```python
from build123d import *

# Parameters (mm, degrees)
SKETCH1_R              = 1.651
SKETCH1_R_2            = 1.8415
SKETCH1_R_3            = 1.905
SKETCH1_R_4            = 3.175
SKETCH1_R_5            = 1.315256363
SKETCH1_R_6            = 1.5621
SKETCH1_R_7            = 5.08
SKETCH1_R_8            = 2.2479
BOSS_EXTRUDE1_DEPTH    = 6.35
FILLET_OUTER_CORNERS_R = 12.7
FILLET_INNER_CORNERS_R = 6.35
SKETCH2_R              = 5.08
CUT_EXTRUDE1_DEPTH     = 220.86103505


with BuildPart() as part:
    # Sketch1 → Boss-Extrude1 (new body)
    with BuildSketch(Plane(origin=(0, 0, 0), x_dir=(1, 0, 0), z_dir=(0, 1, 0))):
        with BuildLine():
            Line((-142.875, 95.25), (-41.275, 95.25))
            Line((-41.275, 95.25), (-41.275, 139.7))
            Line((-41.275, 139.7), (41.275, 139.7))
            Line((41.275, 139.7), (41.275, 95.25))
            Line((41.275, 95.25), (142.875, 95.25))
            Line((142.875, 95.25), (170.571792564, 95.25))
            ThreePointArc((170.571792564, 95.25), (166.994880438, 0), (170.571792564, -95.25))
            Line((170.571792564, -95.25), (142.875, -95.25))
            Line((142.875, -95.25), (41.275, -95.25))
            Line((41.275, -95.25), (41.275, -139.7))
            Line((41.275, -139.7), (-41.275, -139.7))
            Line((-41.275, -139.7), (-41.275, -95.25))
            Line((-41.275, -95.25), (-142.875, -95.25))
            Line((-142.875, -95.25), (-170.571792564, -95.25))
            ThreePointArc((-170.571792564, -95.25), (-166.994880438, 0), (-170.571792564, 95.25))
            Line((-170.571792564, 95.25), (-142.875, 95.25))
        make_face()
        with Locations(Location((-107.696, 77.978, 0), (0, 0, 270))):
            Circle(SKETCH1_R, mode=Mode.SUBTRACT)
        with Locations(Location((-107.696, 65.278, 0), (0, 0, 270))):
            Circle(SKETCH1_R, mode=Mode.SUBTRACT)
        with Locations(Location((-107.696, 52.578, 0), (0, 0, 270))):
            Circle(SKETCH1_R, mode=Mode.SUBTRACT)
        with Locations(Location((-76.454, 77.978, 0), (0, 0, 90))):
            Circle(SKETCH1_R, mode=Mode.SUBTRACT)
        with Locations(Location((-76.454, 65.278, 0), (0, 0, 90))):
            Circle(SKETCH1_R, mode=Mode.SUBTRACT)
        with Locations(Location((-76.454, 52.578, 0), (0, 0, 90))):
            Circle(SKETCH1_R, mode=Mode.SUBTRACT)
        with Locations(Location((76.454, 52.578, 0), (0, 0, 270))):
            Circle(SKETCH1_R, mode=Mode.SUBTRACT)
        with Locations(Location((107.696, 52.578, 0), (0, 0, 90))):
            Circle(SKETCH1_R, mode=Mode.SUBTRACT)
        with Locations(Location((76.454, 65.278, 0), (0, 0, 270))):
            Circle(SKETCH1_R, mode=Mode.SUBTRACT)
        with Locations(Location((107.696, 65.278, 0), (0, 0, 90))):
            Circle(SKETCH1_R, mode=Mode.SUBTRACT)
        with Locations(Location((76.454, 77.978, 0), (0, 0, 270))):
            Circle(SKETCH1_R, mode=Mode.SUBTRACT)
        with Locations(Location((107.696, 77.978, 0), (0, 0, 90))):
            Circle(SKETCH1_R, mode=Mode.SUBTRACT)
        with Locations(Location((76.454, -52.578, 0), (0, 0, 90))):
            Circle(SKETCH1_R, mode=Mode.SUBTRACT)
        with Locations(Location((107.696, -52.578, 0), (0, 0, 270))):
            Circle(SKETCH1_R, mode=Mode.SUBTRACT)
        with Locations(Location((107.696, -65.278, 0), (0, 0, 270))):
            Circle(SKETCH1_R, mode=Mode.SUBTRACT)
        with Locations(Location((76.454, -65.278, 0), (0, 0, 90))):
            Circle(SKETCH1_R, mode=Mode.SUBTRACT)
        with Locations(Location((107.696, -77.978, 0), (0, 0, 270))):
            Circle(SKETCH1_R, mode=Mode.SUBTRACT)
        with Locations(Location((76.454, -77.978, 0), (0, 0, 90))):
            Circle(SKETCH1_R, mode=Mode.SUBTRACT)
        with Locations(Location((-76.454, -52.578, 0), (0, 0, 270))):
            Circle(SKETCH1_R, mode=Mode.SUBTRACT)
        with Locations(Location((-107.696, -52.578, 0), (0, 0, 90))):
            Circle(SKETCH1_R, mode=Mode.SUBTRACT)
        with Locations(Location((-76.454, -65.278, 0), (0, 0, 270))):
            Circle(SKETCH1_R, mode=Mode.SUBTRACT)
        with Locations(Location((-107.696, -65.278, 0), (0, 0, 90))):
            Circle(SKETCH1_R, mode=Mode.SUBTRACT)
        with Locations(Location((-76.454, -77.978, 0), (0, 0, 270))):
            Circle(SKETCH1_R, mode=Mode.SUBTRACT)
        with Locations(Location((-107.696, -77.978, 0), (0, 0, 90))):
            Circle(SKETCH1_R, mode=Mode.SUBTRACT)
        with Locations(Location((155.575, 0, 0), (0, 0, 270))):
            Circle(SKETCH1_R_2, mode=Mode.SUBTRACT)
        with Locations(Location((-27.94, -128.27, 0), (0, 0, 270))):
            Circle(SKETCH1_R_3, mode=Mode.SUBTRACT)
        with Locations(Location((27.94, -128.27, 0), (0, 0, 270))):
            Circle(SKETCH1_R_3, mode=Mode.SUBTRACT)
        with Locations(Location((-27.94, -41.91, 0), (0, 0, 90))):
            Circle(SKETCH1_R_3, mode=Mode.SUBTRACT)
        with Locations(Location((27.94, -41.91, 0), (0, 0, 90))):
            Circle(SKETCH1_R_3, mode=Mode.SUBTRACT)
        with Locations(Location((0, 0, 0), (0, 0, 270))):
            Circle(SKETCH1_R_2, mode=Mode.SUBTRACT)
        with Locations(Location((-122.311792564, 69.85, 0), (0, 0, 270))):
            Circle(SKETCH1_R_4, mode=Mode.SUBTRACT)
        with Locations(Location((-61.838207436, 69.85, 0), (0, 0, 90))):
            Circle(SKETCH1_R_4, mode=Mode.SUBTRACT)
        with Locations(Location((-61.838207436, -69.85, 0), (0, 0, 270))):
            Circle(SKETCH1_R_4, mode=Mode.SUBTRACT)
        with Locations(Location((-122.311792564, -69.85, 0), (0, 0, 90))):
            Circle(SKETCH1_R_4, mode=Mode.SUBTRACT)
        with Locations(Location((61.838207436, -69.85, 0), (0, 0, 90))):
            Circle(SKETCH1_R_4, mode=Mode.SUBTRACT)
        with Locations(Location((122.311792564, -69.85, 0), (0, 0, 270))):
            Circle(SKETCH1_R_4, mode=Mode.SUBTRACT)
        with Locations(Location((61.838207436, 69.85, 0), (0, 0, 270))):
            Circle(SKETCH1_R_4, mode=Mode.SUBTRACT)
        with Locations(Location((122.311792564, 69.85, 0), (0, 0, 90))):
            Circle(SKETCH1_R_4, mode=Mode.SUBTRACT)
        with Locations(Location((149.480692766, -14.9479, 0), (0, 0, 270))):
            Circle(SKETCH1_R_5, mode=Mode.SUBTRACT)
        with Locations(Location((121.464492766, -14.9479, 0), (0, 0, 270))):
            Circle(SKETCH1_R_6, mode=Mode.SUBTRACT)
        with Locations(Location((116.586, -45.9486, 0), (0, 0, 270))):
            Circle(SKETCH1_R_6, mode=Mode.SUBTRACT)
        with Locations(Location((164.9222, -38.4556, 0), (0, 0, 270))):
            Circle(SKETCH1_R_6, mode=Mode.SUBTRACT)
        with Locations(Location((164.9222, 36.6776, 0), (0, 0, 270))):
            Circle(SKETCH1_R_6, mode=Mode.SUBTRACT)
        with Locations(Location((116.586, 36.6776, 0), (0, 0, 270))):
            Circle(SKETCH1_R_6, mode=Mode.SUBTRACT)
        with Locations(Location((0, -92.075, 0), (0, 0, 270))):
            Circle(SKETCH1_R_3, mode=Mode.SUBTRACT)
        with Locations(Location((0, 92.075, 0), (0, 0, 270))):
            Circle(SKETCH1_R_3, mode=Mode.SUBTRACT)
        with Locations(Location((-61.838207436, -39.878, 0), (0, 0, 270))):
            Circle(SKETCH1_R_7, mode=Mode.SUBTRACT)
        with Locations(Location((-122.311792564, -39.878, 0), (0, 0, 270))):
            Circle(SKETCH1_R_7, mode=Mode.SUBTRACT)
        with Locations(Location((61.838207436, -39.878, 0), (0, 0, 90))):
            Circle(SKETCH1_R_7, mode=Mode.SUBTRACT)
        with Locations(Location((62.026925824, -8.128150569, 0), (0, 0, 270))):
            Circle(SKETCH1_R_8, mode=Mode.SUBTRACT)
        with Locations(Location((64.176925824, 48.924363993, 0), (0, 0, 270))):
            Circle(SKETCH1_R_8, mode=Mode.SUBTRACT)
        with Locations(Location((64.176925824, 55.924363993, 0), (0, 0, 270))):
            Circle(SKETCH1_R_8, mode=Mode.SUBTRACT)
        with Locations(Location((-33.323074176, 55.924363993, 0), (0, 0, 270))):
            Circle(SKETCH1_R_8, mode=Mode.SUBTRACT)
        with Locations(Location((-33.323074176, 48.924363993, 0), (0, 0, 270))):
            Circle(SKETCH1_R_8, mode=Mode.SUBTRACT)
        with Locations(Location((-39.573074176, 0.761849431, 0), (0, 0, 270))):
            Circle(SKETCH1_R_8, mode=Mode.SUBTRACT)
        with Locations(Location((-84.023074176, 0.761849431, 0), (0, 0, 270))):
            Circle(SKETCH1_R_8, mode=Mode.SUBTRACT)
        with Locations(Location((-128.473074176, 0.761849431, 0), (0, 0, 270))):
            Circle(SKETCH1_R_8, mode=Mode.SUBTRACT)
    extrude(amount=BOSS_EXTRUDE1_DEPTH)

    # Fillet_Outer_Corners
    fillet_outer_corners_edges = [part.edges().sort_by_distance(p)[0] for p in [
        (-170.571792564, 3.175, 95.25),
        (-170.571792564, 3.175, -95.25),
        (-41.275, 3.175, -139.7),
        (41.275, 3.175, -139.7),
        (170.571792564, 3.175, -95.25),
        (170.571792564, 3.175, 95.25),
        (41.275, 3.175, 139.7),
        (-41.275, 3.175, 139.7),
    ]]
    fillet(fillet_outer_corners_edges, radius=FILLET_OUTER_CORNERS_R)

    # Fillet_Inner_Corners
    fillet_inner_corners_edges = [part.edges().sort_by_distance(p)[0] for p in [
        (-41.275, 3.175, -95.25),
        (41.275, 3.175, -95.25),
        (41.275, 3.175, 95.25),
        (-41.275, 3.175, 95.25),
    ]]
    fillet(fillet_inner_corners_edges, radius=FILLET_INNER_CORNERS_R)

    # Sketch2 → Cut-Extrude1 (cut, through all)
    with BuildSketch(Plane(origin=(0, 6.35, 0), x_dir=(1, 0, 0), z_dir=(0, 1, 0))):
        with Locations(Location((-61.838207436, 39.878, 0), (0, 0, 90))):
            Circle(SKETCH2_R)
    extrude(amount=-CUT_EXTRUDE1_DEPTH, mode=Mode.SUBTRACT)


solid = part.part
```
Source: CAD feature listing. Evaluate the final solid. Frame: model axes, mm. Coordinates: 2 decimals unless noted, no trailing zeros. Loops run counter-clockwise (first coordinate to the right, second up) from the corner with the lowest first, then second, coordinate; pieces in that order, holes last. Notation, with made-up numbers: M 33,13.25 L 78,13.25 A19 ccw 78,18.25 Z; hole C 53.25,6 d1. An arc over 180 degrees is marked long. Use CSV: the item, a comma, the result in double quotes.
(1) Cut plane B-B on y = 5.25. Give the number of separate pieces and of enclosed holes in the cut face, and give its area (3 significant figures).
Answers follow:
separate pieces,"1"
enclosed holes,"58"
area,"70,100 mm²"
(2) Contact query for a flat-ended pin moving along its axis: pin 1 (3 mm diameter, centred on x = 107.696, z = 77.978, fed in from +Y). Output: stop coordinate, or through.
Answers follow:
pin 1,"through"
(3) Line query: line 1 (X direction, y = 4, z = 67); line 2 (X direction, y = 5, z = -56); line 3 (Z direction, x = 60.5, y = 2.75). Output: solid intervals per line, ascending. Write a range as [from, to].
Answers follow:
line 1,"[-168.76, -123.71], [-120.91, -63.24], [-60.44, 60.44], [63.24, 120.91], [123.71, 168.76]"
line 2,"[-168.23, -35.57], [-31.08, 61.93], [66.42, 168.23]"
line 3,"[-95.25, -72.73], [-66.97, 6.48], [9.78, 34.98], [44.78, 66.97], [72.73, 95.25]"
(4) Draft query along X for faces 1 (the face through (-124.26, 3.13, 44.57)), 2 (the face through (2, 6.35, -2)), 3 (the face through (-66.345, 3.131, 42.222)), 4 (the face through (37.456, 3.219, 136.078)). Return one class per face: pulls with the +X half, pulls with the -X half, needs draft (parallel to the pull), parting line crosses it, or undercut.
Answers follow:
face 1,"undercut"
face 2,"needs draft"
face 3,"undercut"
face 4,"pulls with the +X half"
(5) Cut plane A-A on z = -119.5. Return loops of the section in (x, y) (3 decimals), and give its area (3 significant figures).
Answers follow:
outline,"M -41.275,0 L 41.275,0 L 41.275,6.35 L -41.275,6.35 Z"
area,"524 mm²"
